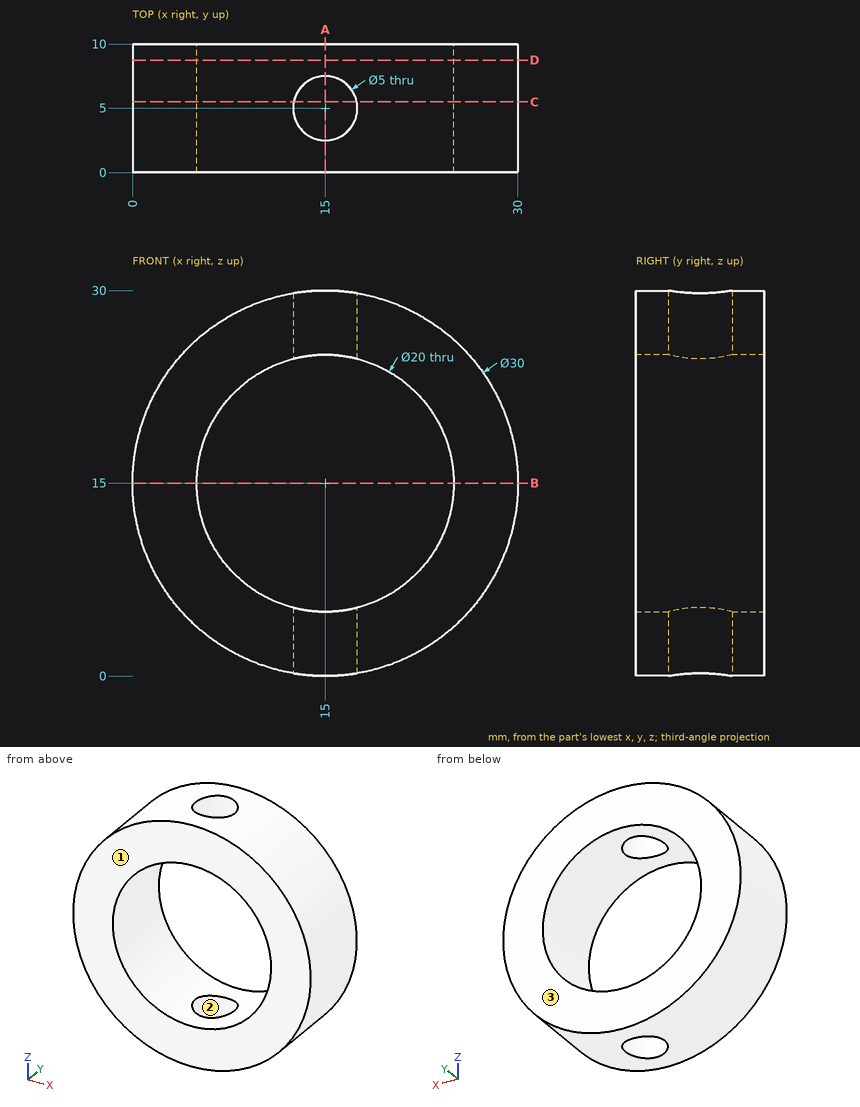
Part print with two shaded views. Sizes in mm from the minimum x, y, z corner. Round coordinates to 2 decimals unless told otherwise and drop trailing zeros. Loops run counter-clockwise (first coordinate to the right, second up) from the corner with the lowest first, then second, coordinate; pieces in that order, holes last. Notation, with made-up numbers: M -3,76 L 7,76 A27 cw 7,100 Z; hole C 38.5,-22.75 d3. An arc over 180 degrees is marked long. Return JSON: item names as keys, results as strings. Group by question number.
(1) Wall check: probe 1 along X at (y, z) = (5, 15); probe 2 along Z at (x, y) = (10, 4.5); probe 3 along X at (y, z) = (1, 11). Give the ranges that are in metal, low to high. Write a range as [from, to].
(2) Saw through at D-D, the plane y = 8.75. List the corners of the cut face in (x, z), and give its area (3 significant figures).
(3) Saw through at C-C, the plane y = 5.5. List the corners of the cut face in (x, z), and give its area (3 significant figures).
(4) Saw through at B-B, the plane z = 15. List the corners of the cut face in (x, y).
(5) Mould opens along Y. For the marked faces 1, 2 and 3 say: +Y half, -Y half, draft (parallel to the pull), parting line (faces both ways), or undercut.
(6) Drop flat-ended pins along their axis: P1, Ø4, axis at y = 4.5, z = 12.5, coming from the +X side; P2, Ø4, axis at x = 22, y = 3, coming from the +Z side; P3, Ø5, axis at y = 4.5, z = 5, coming from the -X side. Give the stop position or say it passes through.
(7) Saw through at A-A, the plane x = 15. List the corners of the cut face in (y, z), and give its area (3 significant figures).
Answer list:
{
 "1": {"probe 1": "[0, 5], [25, 30]", "probe 2": "[0.86, 6.34], [23.66, 29.14]", "probe 3": "[0.54, 5.83], [24.17, 29.46]"},
 "2": {"outline": "C 15,15 d30; hole C 15,15 d20", "area": "393 mm2"},
 "3": {"outline": "M 12.55,0.2 L 12.55,5.3 A10 cw 12.55,24.7 L 12.55,29.8 A15 ccw Z; M 17.45,0.2 A15 ccw 17.45,29.8 L 17.45,24.7 A10 cw 17.45,5.3 Z", "area": "343 mm2"},
 "4": {"outline": "M 0,0 L 5,0 L 5,10 L 0,10 Z; M 25,0 L 30,0 L 30,10 L 25,10 Z"},
 "5": {"face 1": "-Y half", "face 2": "undercut", "face 3": "+Y half"},
 "6": {"P1": "x = 29.99", "P2": "z = 29.14", "P3": "x = 2.01"},
 "7": {"outline": "M 0,0 L 2.5,0 L 2.5,5 L 0,5 Z; M 0,25 L 2.5,25 L 2.5,30 L 0,30 Z; M 7.5,0 L 10,0 L 10,5 L 7.5,5 Z; M 7.5,25 L 10,25 L 10,30 L 7.5,30 Z", "area": "50.0 mm2"}
}
